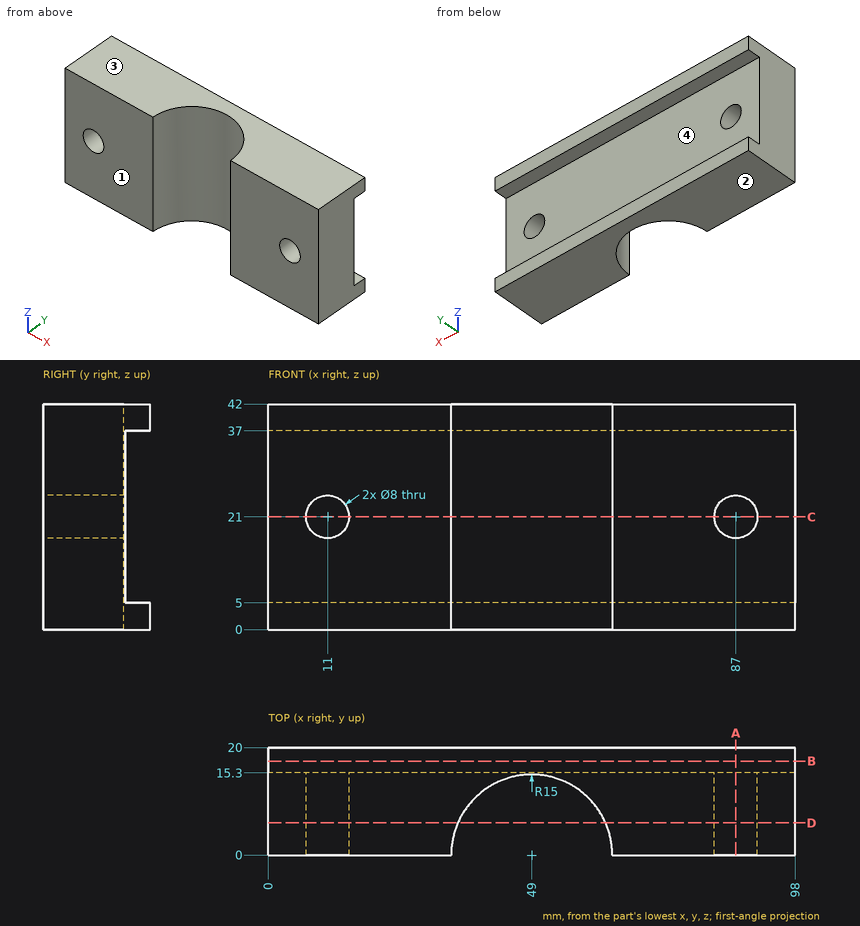
Here's the drawing with two shaded views (mm, measured from the low corner). I have some questions. Coordinates: 2 decimals unless noted, no trailing zeros. Order: outer loops, then holes, each group sorted by start corner. A loop starts at its lowest first (then second) coordinate and runs counter-clockwise, first axis right, second up. Notation, with made-up numbers: M -18,83 L 5,83 A30 ccw 5,120 Z; hole C 3.25,13.25 d8. An arc over 180 degrees is marked long. Answer as CSV lines item,"result".
Item 1: If I drill on line 1 (Z direction, x = 87, y = 7.5); line 2 (X direction, y = 12.25, z = 21); line 3 (X direction, y = 8, z = 21), over which ranges is the centre line in solid material (lowest first)?
Results found:
line 1,"0 to 17, 25 to 42"
line 2,"0 to 7, 15 to 40.34, 57.66 to 83, 91 to 98"
line 3,"0 to 7, 15 to 36.31, 61.69 to 83, 91 to 98"
Item 2: For pin 1 (8 mm diameter, centred on x = 51.5, z = 16.5, fed in from -Y); pin 2 (5 mm diameter, centred on x = 87, z = 21, fed in from +Y); pin 3 (16 mm diameter, centred on x = 55.5, z = 15.5, fed in from +Y), each with a flat end and sliding along its axis, tell me the tip position at first contact or that it passes through.
Results found:
pin 1,"y = 13.52"
pin 2,"through"
pin 3,"y = 15.3"
Item 3: Imagine slicing it at A-A on x = 87. Write out the boundary of the cut face in (y, z), plus the area to 3 significant figures.
Results found:
outline,"M 0,0 L 20,0 L 20,5 L 15.3,5 L 15.3,17 L 0,17 Z; M 0,25 L 15.3,25 L 15.3,37 L 20,37 L 20,42 L 0,42 Z"
area,"567 mm2"
Item 4: We'd pull the mould along Z, two halves only. Please class the marked faces 1, 2, 3 and 4: +Z half, -Z half, draft (parallel to the pull), parting line (faces both ways), or undercut.
Results found:
face 1,"draft"
face 2,"-Z half"
face 3,"+Z half"
face 4,"undercut"
Item 5: Imagine slicing it at D-D on y = 6. Write out the boundary of the cut face in (x, z).
Results found:
outline,"M 0,0 L 35.25,0 L 35.25,42 L 0,42 Z; M 62.75,0 L 98,0 L 98,42 L 62.75,42 Z; hole C 11,21 d8; hole C 87,21 d8"
Item 6: Imagine slicing it at C-C on z = 21. Write out the boundary of the cut face in (x, y), plus the area to 3 significant figures.
Results found:
outline,"M 0,0 L 7,0 L 7,15.3 L 0,15.3 Z; M 15,0 L 34,0 A15 cw 64,0 L 83,0 L 83,15.3 L 15,15.3 Z; M 91,0 L 98,0 L 98,15.3 L 91,15.3 Z"
area,"901 mm2"
Item 7: Imagine slicing it at B-B on y = 17.5. Write out the boundary of the cut face in (x, z).
Results found:
outline,"M 0,0 L 98,0 L 98,5 L 0,5 Z; M 0,37 L 98,37 L 98,42 L 0,42 Z"
